```python
from build123d import *

# Parameters (mm, degrees)
SKETCH1_W           = 65
SKETCH1_H           = 400
SKETCH1_R           = 2.54
SKETCH1_R_2         = 12.7
SKETCH1_R_3         = 2.75
BOSS_EXTRUDE1_DEPTH = 10


with BuildPart() as part:
    # Sketch1 → Boss-Extrude1 (new body)
    with BuildSketch(Plane.XY):
        with Locations((0, -171.425)):
            Rectangle(SKETCH1_W, SKETCH1_H)
        with Locations((-23.5712, 23.5712)):
            Circle(SKETCH1_R, mode=Mode.SUBTRACT)
        with Locations((23.5712, 23.5712)):
            Circle(SKETCH1_R, mode=Mode.SUBTRACT)
        with Locations((23.5712, -23.5712)):
            Circle(SKETCH1_R, mode=Mode.SUBTRACT)
        with Locations((-23.5712, -23.5712)):
            Circle(SKETCH1_R, mode=Mode.SUBTRACT)
        Circle(SKETCH1_R_2, mode=Mode.SUBTRACT)
        with Locations((18, 16)):
            Circle(SKETCH1_R_3, mode=Mode.SUBTRACT)
        with Locations((-18, 16)):
            Circle(SKETCH1_R_3, mode=Mode.SUBTRACT)
        with Locations((18, -106)):
            Circle(SKETCH1_R_3, mode=Mode.SUBTRACT)
        with Locations((-18, -106)):
            Circle(SKETCH1_R_3, mode=Mode.SUBTRACT)
    extrude(amount=BOSS_EXTRUDE1_DEPTH)


solid = part.part
```
Part model, mm, in its own coordinate system. Give positions to 0.01 mm unless a question says otherwise; leave off trailing zeros. Write each loop counter-clockwise with the first axis right and the second up, starting at its lowest first coordinate (ties: lowest second). Pieces come first, ordered by that corner, then holes. Notation, with made-up numbers: M 62,13 L 80,13 A23 ccw 80,28 Z; hole C 67,28 d6. An arc over 180 degrees is marked long. Use CSV: the item, a comma, the result in double quotes.
Item 1: Drill centre lines: probe 1 along Y at (x, z) = (18, 7.25) (3 decimals); probe 2 along Y at (x, z) = (24, 7) (3 decimals); probe 3 along Y at (x, z) = (0, 6.5) (3 decimals). Where is each one in solid material? Low to high.
Taken from the geometry:
probe 1,"y = -371.425 to -108.75, -103.25 to 13.25, 18.75 to 28.575"
probe 2,"y = -371.425 to -26.075, -21.068 to 21.068, 26.075 to 28.575"
probe 3,"y = -371.425 to -12.7, 12.7 to 28.575"
Item 2: Pull direction Y, two halves, no side cores. Call faces 1 (the face through (0, 28.575, 5)), 2 (the face through (-2.75, -12.4, 4.93)), 3 (the face through (0, -371.425, 5)): +Y half, -Y half, draft (parallel to the pull), parting line (faces both ways), or undercut.
Taken from the geometry:
face 1,"+Y half"
face 2,"undercut"
face 3,"-Y half"
Item 3: Pin check, flat tip, straight feed: P1, Ø4, axis at x = -23.57, y = -23.57, coming from the +Z side. Stop position of the tip, or through.
Taken from the geometry:
P1,"passes through"
Item 4: Slice it at A-A on y = 0. Write the cut outline in (x, z).
Taken from the geometry:
outline,"M -32.5,0 L -12.7,0 L -12.7,10 L -32.5,10 Z; M 12.7,0 L 32.5,0 L 32.5,10 L 12.7,10 Z"
Item 5: Slice it at C-C on z = 4. State how many separate pieces and enclosed holes the cut face has, plus the area to 3 significant figures.
Taken from the geometry:
separate pieces,"1"
enclosed holes,"9"
area,"25,300 mm²"
Item 6: Slice it at B-B on x = 0. Write the cut outline in (y, z) (3 decimals), plus the area to 3 significant figures.
Taken from the geometry:
outline,"M -371.425,0 L -12.7,0 L -12.7,10 L -371.425,10 Z; M 12.7,0 L 28.575,0 L 28.575,10 L 12.7,10 Z"
area,"3,750 mm²"
